Geometry check sheet. Reference: drawing and pictorial views, mm from the part's lowest x, y, z. Coordinates: 2 decimals unless noted, no trailing zeros. Write each loop counter-clockwise with the first axis right and the second up, starting at its lowest first coordinate (ties: lowest second). Pieces come first, ordered by that corner, then holes. Notation, with made-up numbers: M 24.5,48.5 L 75.5,48.5 A8 cw 75.5,58.5 Z; hole C 7,42.25 d10. An arc over 180 degrees is marked long. One line per item, written item: value.
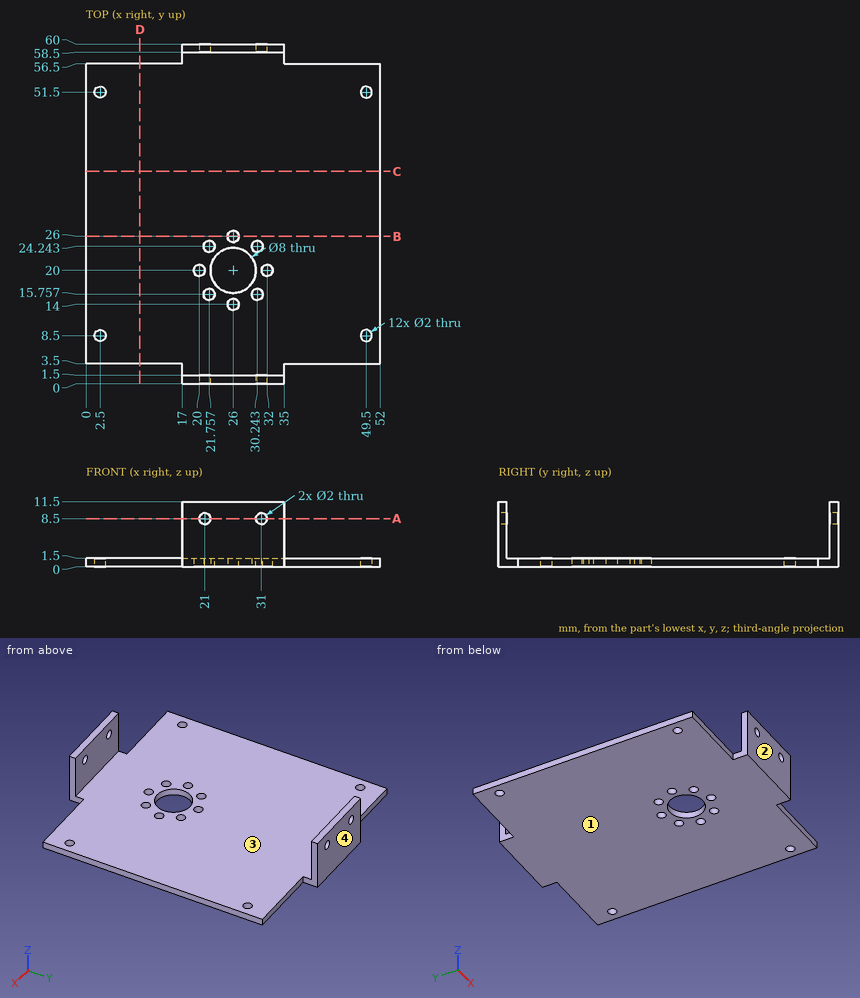
Item 1: Cross-section at A-A, the plane z = 8.5. Enter the section's corners in (x, y).
The answers:
outline: M 17,0 L 20,0 L 20,1.5 L 17,1.5 Z; M 17,58.5 L 20,58.5 L 20,60 L 17,60 Z; M 22,0 L 30,0 L 30,1.5 L 22,1.5 Z; M 22,58.5 L 30,58.5 L 30,60 L 22,60 Z; M 32,0 L 35,0 L 35,1.5 L 32,1.5 Z; M 32,58.5 L 35,58.5 L 35,60 L 32,60 Z
Item 2: Cross-section at B-B, the plane y = 26. Enter the section's corners in (x, z).
The answers:
outline: M 0,0 L 25,0 L 25,1.5 L 0,1.5 Z; M 27,0 L 52,0 L 52,1.5 L 27,1.5 Z
Item 3: Cross-section at C-C, the plane y = 37.5. Enter the section's corners in (x, z).
The answers:
outline: M 0,0 L 52,0 L 52,1.5 L 0,1.5 Z
Item 4: Scan lines: line 1 (X direction, y = 51.5, z = 0.75); line 2 (X direction, y = 59.65, z = 8.5); line 3 (Y direction, x = 49.5, z = 0.8). Record each from-to range of solid material in increasing order.
The answers:
line 1: x = 0 to 1.5, 3.5 to 48.5, 50.5 to 52
line 2: x = 17 to 20, 22 to 30, 32 to 35
line 3: y = 3.5 to 7.5, 9.5 to 50.5, 52.5 to 56.5
Item 5: Go/stop test with flat-tipped pins: P1, Ø3, axis at y = 1, z = 6, coming from the +X side; P2, Ø3, axis at x = 49.5, y = 51.5, coming from the +Z side; P3, Ø1.8, axis at y = 58, z = 4.5, coming from the -X side. Record where each tip stops, or that it passes through.
The answers:
P1: stops at x = 35
P2: stops at z = 1.5
P3: stops at x = 17
Item 6: Cross-section at D-D, the plane x = 9.5. Enter the section's corners in (y, z).
The answers:
outline: M 3.5,0 L 56.5,0 L 56.5,1.5 L 3.5,1.5 Z
Item 7: Draft check along Y on the marked faces 1, 2, 3 and 4. Enter one of: released by +Y, released by -Y, zero draft, split by the parting line, or undercut.
The answers:
face 1: zero draft
face 2: released by -Y
face 3: undercut
face 4: released by +Y
